```python
from build123d import *

# Parameters (mm, degrees)
F2_R     = 17.3084147979
F2_R_2   = 9.8858681408
F2_R_3   = 11.8408403521
F2_R_4   = 33.563848705
F3_DEPTH = 77.9319693274
F4_W     = 15.939405188
F4_H     = 86.4525958896
F5_DEPTH = 77.9319694274


with BuildPart() as f1:
    # F0 (on Front) → F1 (revolve)
    with BuildSketch(Plane.XZ):
        Polygon((23.8796671181, -76.2), (77.9309693274, -17.4196016418), (54.0513022093, 58.7803983582), (-23.8796671181, 76.2), (-77.9309693274, 17.4196016418), (-54.0513022093, -58.7803983582), align=None)
    revolve(axis=Axis((15.0858175456, 0, 67.4901991791), (0.9759168522, 0, -0.2181428378)))

    # F2 (on Right) → F3 (cut, through all)
    with BuildSketch(Plane.YZ):
        with Locations((77.9518336058, 37.3855829239)):
            Circle(F2_R)
        with Locations((31.3565693796, 10.4093803093)):
            Circle(F2_R_2)
        with Locations((-56.9291785359, 19.605813548)):
            Circle(F2_R_3)
        with Locations((-67.351795733, 102.3737117648)):
            Circle(F2_R_4)
    extrude(amount=-F3_DEPTH, mode=Mode.SUBTRACT)

    # F4 (on Right) → F5 (cut, through all)
    with BuildSketch(Plane.YZ):
        with Locations((-33.2528958097, 43.2262979448)):
            Rectangle(F4_W, F4_H)
    extrude(amount=-F5_DEPTH, mode=Mode.SUBTRACT)


solid = f1.part
```
Geometry: final body of the model. Coordinates: model frame, mm. A direction names the side the tool comes from. Coordinates: 2 decimals unless noted, no trailing zeros. Answer as CSV lines item,"result". Start each with the question number.
Q1. Mould query, pull axis Y, two halves, no side actions, for faces 1 (the cylindrical face through (-26.35, 60.66, 38.15)), 2 (the flat face through (-29, -41.223, 40)), 3 (the conical face through (94.554, -70.789, 65.834)). Classes: released by +Y, released by -Y, zero draft, split by the parting line, or undercut.
Q2. Reachability of faces 4 (the conical face through (57.975, 3.317, 47.111)), 5 (the flat face through (0, 31, 11)) from +Z, -Z, +X, -X, +Y, -Y: full face, straight path, thin tool, end or side. Return the list, or none.
Q3. Line query: line 1 (Y direction, x = -3, z = 37); line 2 (Y direction, x = -58.5, z = 68); line 3 (Z direction, x = 28.5, y = -44). Output: solid intervals per line, ascending. Write a range as from..to.
Q4. Cut plane A-A on x = -9.5. Count the separate pieces of the cut face and the enclosed holes in it, then the cut area to 3 significant figures.
Q5. Pin query (flat end, axial travel): P1, Ø16, axis at y = 31.36, z = 10.41, coming from the -X side; P2, Ø14, axis at x = -24, y = -31.5, coming from the -Z side; P3, Ø1.5, axis at x = -38.5, y = -34, coming from the +Z side. Return the tip coordinate at first contact, or that it passes through.
Findings below:
1,face 1,"undercut"
1,face 2,"undercut"
1,face 3,"split by the parting line"
2,face 4,"+X"
2,face 5,"-X"
3,line 1,"y = -134.14..-41.22, -25.28..60.65, 95.26..134.14"
3,line 2,"y = -81.42..-53.19, 53.19..81.42"
3,line 3,"z = -65.71..198.85"
4,separate pieces,"1"
4,enclosed holes,"4"
4,area,"51,100 mm2"
5,P1,"stops at x = 0"
5,P2,"stops at z = -63.97"
5,P3,"stops at z = 158"
